For this review, take the finished solid that the model builds, in its own axes (mm). Give positions to 0.01 mm unless a question says otherwise; leave off trailing zeros. Loops run counter-clockwise (first coordinate to the right, second up) from the corner with the lowest first, then second, coordinate; pieces in that order, holes last.
Autodesk Inventor part; units mm, degrees
ref_plane "YZ Plane" through (0, 0, 0) normal (1, 0, 0) x (0, 1, 0)
ref_plane "XZ Plane" through (0, 0, 0) normal (0, 1, 0) x (-1, 0, 0)
ref_plane "XY Plane" through (0, 0, 0) normal (0, 0, 1) x (1, 0, 0)
sketch "Szkic1" plane through (0, 0, 0) normal (0, 1, 0) x (-1, 0, 0)
  line L0 (40, -20) -> (-40, -20)
  line L1 (-40, -20) -> (-40, 20)
  line L2 (-40, 20) -> (40, 20)
  line L3 (40, 20) -> (40, -20)
  line L4 (40, -20) -> (-40, 20) construction
  line L5 (-40, -20) -> (40, 20) construction
  point P0 (0, 0)
  dimension "d0" = 80
  dimension "d1" = 40
extrude "Wyciągnięcie proste1" add sketch "Szkic1" along normal blind 3
sketch "Szkic2" plane through (0, 3, 0) normal (0, 1, 0) x (1, 0, 0)
  line L0 (40, 20) -> (-40, 20)
  line L1 (34, 14) -> (34, -14)
  line L2 (-34, -14) -> (-34, 14)
  line L3 (-34, 14) -> (-6, 14)
  line L4 (-6, 14) -> (-6, -14)
  line L5 (-6, -14) -> (-34, -14)
  line L6 (-34, -14) -> (-34, 14)
  line L7 (34, 14) -> (6, 14)
  line L8 (6, 14) -> (6, -14)
  line L9 (6, -14) -> (34, -14)
  line L10 (34, -14) -> (34, 14)
  line L11 (6, 14) -> (34, -14) construction
  line L12 (34, 14) -> (6, -14) construction
  line L13 (-6, 14) -> (-34, -14) construction
  line L14 (-34, 14) -> (-6, -14) construction
  point P0 (0, 0)
  point P1 (-20, 0)
  point P2 (20, 0)
  dimension "d16" = 6
  dimension "d17" = 12
hole "Otwór1" at (34, 3, -14) at (34, 3, 14) at (-34, 3, 14) at (-34, 3, -14) at (6, 3, 14) at (-6, 3, 14) at (6, 3, -14) at (-6, 3, -14) at (20, 3, 0) at (-20, 3, 0) direction (0, -1, 0) diameter 5 end through all
equation "\"d17\" = 2 * d16"
properties part number "płaskownik"
Q1. Consider section C-C on z = 14. Give the boundary of the cut face in (x, y), plus the area to 3 significant figures.
Answers:
outline: (-40, 0) - (-36.5, 0) - (-36.5, 3) - (-40, 3) - close; (-31.5, 0) - (-8.5, 0) - (-8.5, 3) - (-31.5, 3) - close; (-3.5, 0) - (3.5, 0) - (3.5, 3) - (-3.5, 3) - close; (8.5, 0) - (31.5, 0) - (31.5, 3) - (8.5, 3) - close; (36.5, 0) - (40, 0) - (40, 3) - (36.5, 3) - close
area: 180 mm2
Q2. For probe 1 along X at (y, z) = (1.4, 0); probe 2 along X at (y, z) = (2.3, 14); probe 3 along Z at (x, y) = (34, 1.15), list the stretches that pass through material, from the lowest coordinate up.
Answers:
probe 1: x = -40 to -22.5, -17.5 to 17.5, 22.5 to 40
probe 2: x = -40 to -36.5, -31.5 to -8.5, -3.5 to 3.5, 8.5 to 31.5, 36.5 to 40
probe 3: z = -20 to -16.5, -11.5 to 11.5, 16.5 to 20
Q3. Mouldability with a two-part tool opening along X and no side actions: class faces 1 (the flat face through (40, 1, 0)), 2 (the flat face through (-1, 1, -20)), 3 (the cylindrical face through (-22.48, 1.48, -0.33)), 4 (the cylindrical face through (5.9, 1.5, 11.5)) as +X half, -X half, draft (parallel to the pull), parting line (faces both ways), or undercut.
Answers:
face 1: +X half
face 2: draft
face 3: undercut
face 4: undercut
Q4. Consider section D-D on y = 2. Count the separate pieces of the cut face and the enclosed holes in it, plus the area to 3 significant figures.
Answers:
separate pieces: 1
enclosed holes: 10
area: 3,000 mm2
Q5. For pin 1 Ø4 at (x, z) = (20, 0) entering from -Y, flat-tipped, find the tip position at first contact; note if it passes through.
Answers:
pin 1: passes through
Q6. Consider section A-A on x = -6. Give the boundary of the cut face in (y, z).
Answers:
outline: (0, -20) - (3, -20) - (3, -16.5) - (0, -16.5) - close; (0, -11.5) - (3, -11.5) - (3, 11.5) - (0, 11.5) - close; (0, 16.5) - (3, 16.5) - (3, 20) - (0, 20) - close
Q7. Consider section B-B on x = 20. Give the boundary of the cut face in (y, z).
Answers:
outline: (0, -20) - (3, -20) - (3, -2.5) - (0, -2.5) - close; (0, 2.5) - (3, 2.5) - (3, 20) - (0, 20) - close
